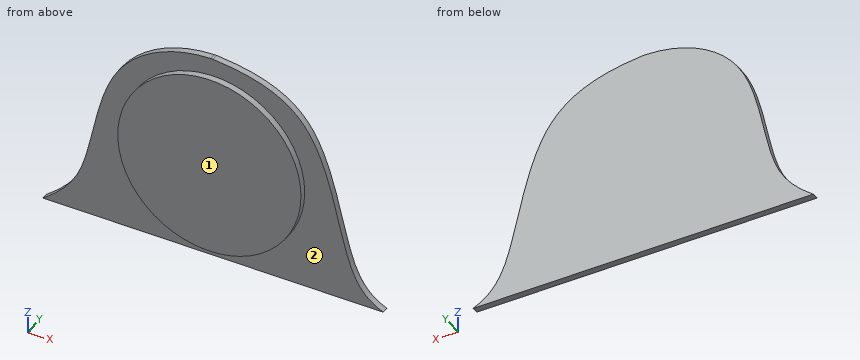
from build123d import *

# Parameters (mm, degrees)
F0_R     = 533.4
F1_DEPTH = 76.2
F2_DEPTH = 38.1


with BuildPart() as f1:
    # F0 (on Front) → F1 (new body)
    with BuildSketch(Plane.XZ):
        Circle(F0_R)
    extrude(amount=F1_DEPTH)

    # F0 (on Front) → F2 (join)
    with BuildSketch(Plane.XZ):
        with BuildLine():
            add(Edge.make_bspline(
                [(0, 636.7163507462), (239.2118357706, 615.8238007368), (646.7304954871, 494.7721182449), (752.2000078985, -358.8744339162), (888.6927709826, -538.11212785), (990.6, -582.4836492538)],
                knots=[0, 0, 0, 0, 0.3511045998, 0.7477812832, 1, 1, 1, 1], degree=3))
            Line((0, 636.7163507462), (-16.1643760611, 636.7163507462))
            add(Edge.make_bspline(
                [(-16.1643760611, 636.7163507462), (-229.7135389785, 634.3414307642), (-676.1585202117, 432.5072199226), (-703.987628904, -342.8286029025), (-907.6178488485, -520.3338171156), (-990.6, -582.4836492538)],
                knots=[0.008772266, 0.008772266, 0.008772266, 0.008772266, 0.3564248173, 0.7365874264, 1, 1, 1, 1], degree=3))
            Line((-990.6, -582.4836492538), (990.6, -582.4836492538))
        make_face()
        Circle(F0_R, mode=Mode.SUBTRACT)
    extrude(amount=F2_DEPTH)


solid = f1.part
Source: CAD feature listing. Evaluate the final solid. Frame: model axes, mm. Face numbers are marked on the shaded views. A direction names the side the tool comes from. Round coordinates to 2 decimals unless told otherwise and drop trailing zeros. Answer as CSV lines item,"result".
Q1. Contact query for flat-ended pins moving along their axis: pin 1 (3 mm diameter, centred on x = 648.5, z = -383.5, fed in from -Y); pin 2 (8 mm diameter, centred on y = -46.5, z = -307.5, fed in from -X); pin 3 (8 mm diameter, centred on x = 576, y = -34.5, fed in from +Z). Output: stop coordinate, or through.
Verdict:
pin 1,"stops at y = -38.1"
pin 2,"stops at x = -438.64"
pin 3,"stops at z = 352.94"
Q2. Reachability of the marked faces 1 and 2 from +Z, -Z, +X, -X, +Y, -Y: full face, straight path, thin tool, end or side. Return the list, or none.
Verdict:
face 1,"+Z, -Z, +X, -X, -Y"
face 2,"-Y"
Q3. Line query: line 1 along Y through (x, z) = (-699, -268.5); line 2 along X through (y, z) = (-19, 489); line 3 along X through (y, z) = (-12, -94.5). Output: solid intervals per line, ascending.
Verdict:
line 1,"y = -38.1 to 0"
line 2,"x = -440.98 to 456.05"
line 3,"x = -708.75 to 726.54"
